CAD build for the part. Positions are in the model's coordinates, mm. A direction names the side the tool comes from. Coordinates: 2 decimals unless noted, no trailing zeros. Write each loop counter-clockwise with the first axis right and the second up, starting at its lowest first coordinate (ties: lowest second). Pieces come first, ordered by that corner, then holes. Notation, with made-up numbers: (12.5, -33) - (68.5, -33) arc R19 cw to (68.5, 1) - close; hole circle Ø7 at (16, 42). An arc over 180 degrees is marked (long way). One line per question, with ' | ' between items. Start each with the question number.
1. Band-saw the part on B-B, the plane x = 0. Write the cut outline in (y, z).
2. Two-plate mould, pull along Y, no slides. Class faces 3 (the cylindrical face through (16.69, 5.26, 2.53)), 4 (the flat face through (8, -4, 5.131)), 5 (the cylindrical face through (10.336, -0.98, 2.529)): +Y half, -Y half, draft (parallel to the pull), parting line (faces both ways), or undercut.
3. Band-saw the part on A-A, the plane y = 0. Write the cut outline in (x, z), then the cut area to 3 significant figures.
4. Flat gauge pins, fed straight in: P1, Ø6, axis at x = -12.7, y = 0, coming from the +Z side; P2, Ø3, axis at x = -3.5, z = 10.5, coming from the -Y side; P3, Ø2, axis at y = -8.5, z = 4, coming from the -X side. Where does each tip first touch, or does it go through?
5. Band-saw the part on D-D, the plane y = -5. Write the cut outline in (x, z), then the cut area to 3 significant figures.
6. Band-saw the part on C-C, the plane z = 12.5. Write the cut outline in (x, y).
7. Which spindle directions (+Z, -Z, +X, -X, +Y, -Y) get a long thin tool onto all of the face, cutting with end or side? Do faces 1 (the cylindrical face through (-1.65, -7.44, 9.51)), 2 (the flat face through (-4.1, 4.1, 0)). Say none if no direction does.
8. Probe line 1 (Y direction, x = 0, z = 8); line 2 (Z direction, x = -16, y = 7); line 3 (Y direction, x = -5, z = 12). List the from-to ranges inside material, lowest first.
from build123d import *

# Parameters (mm, degrees)
F0_R     = 17.5006
F1_DEPTH = 5.1308
F2_R     = 7.62
F2_R_2   = 5.588
F3_DEPTH = 8.89
F4_R     = 5.588
F5_DEPTH = 14.0218
F7_D     = 5.1181


with BuildPart() as f1:
    # F0 (on Top) → F1 (new body)
    with BuildSketch(Plane.XY):
        Circle(F0_R)
    extrude(amount=F1_DEPTH)

    # F2 (on face) → F3 (join)
    with BuildSketch(Plane.XY.offset(5.1308)):
        Circle(F2_R)
        Circle(F2_R_2, mode=Mode.SUBTRACT)
    extrude(amount=F3_DEPTH)

    # F4 (on face) → F5 (cut, through all)
    with BuildSketch(Plane(origin=(0, 0, 0), x_dir=(1, 0, 0), z_dir=(0, 0, -1))):
        Circle(F4_R)
    extrude(amount=-F5_DEPTH, mode=Mode.SUBTRACT)

    # F7 (through all)
    with Locations(Plane.XY.offset(5.1308)):
        with Locations((-12.7, 0), (12.7, 0)):
            Hole(F7_D / 2)


solid = f1.part
Filled in:
1) outline: (-17.5, 0) - (-5.59, 0) - (-5.59, 14.02) - (-7.62, 14.02) - (-7.62, 5.13) - (-17.5, 5.13) - close; (5.59, 0) - (17.5, 0) - (17.5, 5.13) - (7.62, 5.13) - (7.62, 14.02) - (5.59, 14.02) - close
2) face 3: parting line | face 4: draft | face 5: undercut
3) outline: (-17.5, 0) - (-15.26, 0) - (-15.26, 5.13) - (-17.5, 5.13) - close; (-10.14, 0) - (-5.59, 0) - (-5.59, 14.02) - (-7.62, 14.02) - (-7.62, 5.13) - (-10.14, 5.13) - close; (5.59, 0) - (10.14, 0) - (10.14, 5.13) - (7.62, 5.13) - (7.62, 14.02) - (5.59, 14.02) - close; (15.26, 0) - (17.5, 0) - (17.5, 5.13) - (15.26, 5.13) - close | area: 106 mm²
4) P1: stops at z = 5.13 | P2: stops at y = -7.35 | P3: stops at x = -15.81
5) outline: (-16.77, 0) - (-2.5, 0) - (-2.5, 14.02) - (-5.75, 14.02) - (-5.75, 5.13) - (-16.77, 5.13) - close; (2.5, 0) - (16.77, 0) - (16.77, 5.13) - (5.75, 5.13) - (5.75, 14.02) - (2.5, 14.02) - close | area: 204 mm²
6) outline: circle Ø15.24 at (0, 0); hole circle Ø11.18 at (0, 0)
7) face 1: +Z | face 2: -Z, +X, -X, +Y, -Y
8) line 1: y = -7.62 to -5.59, 5.59 to 7.62 | line 2: z = 0 to 5.13 | line 3: y = -5.75 to -2.5, 2.5 to 5.75
